from build123d import *

# Parameters (mm, degrees)
SKETCH1_W           = 30
SKETCH1_H           = 15
BOSS_EXTRUDE1_DEPTH = 2
SKETCH2_W           = 1.2
SKETCH2_H           = 15
BOSS_EXTRUDE2_DEPTH = 12
SKETCH3_W           = 14.4
SKETCH3_H           = 15
SKETCH3_W_2         = 12
SKETCH3_H_2         = 12.6
BOSS_EXTRUDE3_DEPTH = 12
SKETCH4_R           = 2.5
CUT_EXTRUDE1_DEPTH  = 16
SKETCH5_W           = 14.4
SKETCH5_H           = 15
SKETCH5_W_2         = 12
SKETCH5_H_2         = 12.6
BOSS_EXTRUDE4_DEPTH = 12
SKETCH6_R           = 2.5
CUT_EXTRUDE2_DEPTH  = 16


with BuildPart() as part:
    # Sketch1 → Boss-Extrude1 (new body)
    with BuildSketch(Plane(origin=(0, 0, 0), x_dir=(1, 0, 0), z_dir=(0, 1, 0))):
        Rectangle(SKETCH1_W, SKETCH1_H)
    extrude(amount=BOSS_EXTRUDE1_DEPTH)

    # Sketch2 → Boss-Extrude2 (add)
    with BuildSketch(Plane(origin=(0, 2, 0), x_dir=(1, 0, 0), z_dir=(0, 1, 0))):
        Rectangle(SKETCH2_W, SKETCH2_H)
    extrude(amount=BOSS_EXTRUDE2_DEPTH)

    # Sketch3 → Boss-Extrude3 (add)
    with BuildSketch(Plane(origin=(0, 2, 0), x_dir=(1, 0, 0), z_dir=(0, 1, 0))):
        with Locations((7.8, 0)):
            Rectangle(SKETCH3_W, SKETCH3_H)
        with Locations((7.8, 0)):
            Rectangle(SKETCH3_W_2, SKETCH3_H_2, mode=Mode.SUBTRACT)
    extrude(amount=BOSS_EXTRUDE3_DEPTH)

    # Sketch4 → Cut-Extrude1 (cut)
    with BuildSketch(Plane.XY.offset(7.5)):
        with Locations((7.2, 8)):
            Circle(SKETCH4_R)
    extrude(amount=-CUT_EXTRUDE1_DEPTH, mode=Mode.SUBTRACT)

    # Sketch5 → Boss-Extrude4 (add)
    with BuildSketch(Plane(origin=(0, 2, 0), x_dir=(1, 0, 0), z_dir=(0, 1, 0))):
        with Locations((-7.8, 0)):
            Rectangle(SKETCH5_W, SKETCH5_H)
        with Locations((-7.8, 0)):
            Rectangle(SKETCH5_W_2, SKETCH5_H_2, mode=Mode.SUBTRACT)
    extrude(amount=BOSS_EXTRUDE4_DEPTH)

    # Sketch6 → Cut-Extrude2 (cut)
    with BuildSketch(Plane.XY.offset(7.5)):
        with Locations((-7.2, 8)):
            Circle(SKETCH6_R)
    extrude(amount=-CUT_EXTRUDE2_DEPTH, mode=Mode.SUBTRACT)


solid = part.part
Work out the finished part from the listing and answer in its coordinate system (mm). A direction names the side the tool comes from. Round coordinates to 2 decimals unless told otherwise and drop trailing zeros. Loops run counter-clockwise (first coordinate to the right, second up) from the corner with the lowest first, then second, coordinate; pieces in that order, holes last. Notation, with made-up numbers: (10.5, 36.25) - (16.5, 36.25) arc R3 ccw to (16.5, 41.25) - close; hole circle Ø7 at (76, 15.5). An arc over 180 degrees is marked (long way). One line per item, written item: value.
Q1. Straight lines are drawn through the part: probe 1 along X at (y, z) = (8.75, -0.25); probe 2 along Y at (x, z) = (-7.2, -6.75); probe 3 along Z at (x, y) = (-9.75, 10.75). For each, find the intervals that lie inside material, in ascending order.
Check values:
probe 1: -15 to -13.8, -1.8 to 1.8, 13.8 to 15
probe 2: 0 to 5.5, 10.5 to 14
probe 3: -7.5 to -6.3, 6.3 to 7.5
Q2. Each of these flat-tipped pins is pushed along its axis until it touches: pin 1 Ø6 at (x, z) = (5, 1.5) entering from +Y; pin 2 Ø4.5 at (x, y) = (7.2, 8) entering from +Z. Where does it stop, or does it pass through?
Check values:
pin 1: y = 2
pin 2: through
Q3. For faces 4 (the flat face through (0, 7, -7.5)), 5 (the flat face through (8, 2, 0)), determine the directions among +Z, -Z, +X, -X, +Y, -Y from which every point of the face is accessible in a straight line to the end or side of a thin tool.
Check values:
face 4: -Z, +X, -X, +Y, -Y
face 5: +Y
Q4. Find section D-D on x = 3. Give the vertices of the cut face in (y, z).
Check values:
outline: (0, -7.5) - (14, -7.5) - (14, -6.3) - (2, -6.3) - (2, 6.3) - (14, 6.3) - (14, 7.5) - (0, 7.5) - close
Q5. Find section C-C on y = 8. Give the vertices of the cut face in (x, z).
Check values:
outline: (-15, -7.5) - (-9.7, -7.5) - (-9.7, -6.3) - (-13.8, -6.3) - (-13.8, 6.3) - (-9.7, 6.3) - (-9.7, 7.5) - (-15, 7.5) - close; (-4.7, -7.5) - (4.7, -7.5) - (4.7, -6.3) - (1.8, -6.3) - (1.8, 6.3) - (4.7, 6.3) - (4.7, 7.5) - (-4.7, 7.5) - (-4.7, 6.3) - (-1.8, 6.3) - (-1.8, -6.3) - (-4.7, -6.3) - close; (9.7, -7.5) - (15, -7.5) - (15, 7.5) - (9.7, 7.5) - (9.7, 6.3) - (13.8, 6.3) - (13.8, -6.3) - (9.7, -6.3) - close
Q6. Find section B-B on x = 7.2. Give the vertices of the cut face in (y, z), and give its area (3 significant figures).
Check values:
outline: (0, -7.5) - (5.5, -7.5) - (5.5, -6.3) - (2, -6.3) - (2, 6.3) - (5.5, 6.3) - (5.5, 7.5) - (0, 7.5) - close; (10.5, -7.5) - (14, -7.5) - (14, -6.3) - (10.5, -6.3) - close; (10.5, 6.3) - (14, 6.3) - (14, 7.5) - (10.5, 7.5) - close
area: 46.8 mm2
Q7. The mould has two halves that part along X. Classify faces 1 (the flat face through (15, 7, 0)), 2 (the flat face through (-15, 7, 0)), 3 (the flat face through (-11, 8, 6.3)): +X half, -X half, draft (parallel to the pull), parting line (faces both ways), or undercut.
Check values:
face 1: +X half
face 2: -X half
face 3: undercut
Q8. Find section A-A on y = 2.75. Give the vertices of the cut face in (x, z).
Check values:
outline: (-15, -7.5) - (15, -7.5) - (15, 7.5) - (-15, 7.5) - close; hole (-13.8, -6.3) - (-1.8, -6.3) - (-1.8, 6.3) - (-13.8, 6.3) - close; hole (1.8, -6.3) - (13.8, -6.3) - (13.8, 6.3) - (1.8, 6.3) - close
